Work out the finished part from the listing and answer in its coordinate system (mm). A direction names the side the tool comes from. Give positions to 0.01 mm unless a question says otherwise; leave off trailing zeros. Loops run counter-clockwise (first coordinate to the right, second up) from the corner with the lowest first, then second, coordinate; pieces in that order, holes last.
from build123d import *

# Parameters (mm, degrees)
IZIM2_R               = 8.5
KES_EKSTR_ZYON1_DEPTH = 89


with BuildPart() as part:
    # Çizim1 → Döndür1 (revolve)
    with BuildSketch(Plane.XY):
        Polygon((-44, 0), (-44, 12), (-41, 12), (-41, 11), (-40, 11), (-40, 12), (40, 12), (40, 11), (41, 11), (41, 12), (44, 12), (44, 0), align=None)
    revolve(axis=Axis((-44, 0, 0), (1, 0, 0)))

    # Çizim2 → Kes-Ekstrüzyon1 (cut, through all)
    with BuildSketch(Plane(origin=(44, 0, 0), x_dir=(0, 0, -1), z_dir=(1, 0, 0))):
        Circle(IZIM2_R)
    extrude(amount=-KES_EKSTR_ZYON1_DEPTH, mode=Mode.SUBTRACT)


solid = part.part
Item 1: Find section C-C, the plane x = 7.5. Write down the section's boundary in (y, z).
Item 2: Find section D-D, the plane z = 9.75. Write down the section's boundary in (x, y).
Item 3: Flat-ended cylindrical pins translate along their axes: pin 1 Ø8 at (y, z) = (-3.5, 3) entering from -X; pin 2 Ø10 at (x, z) = (-6.5, -5.5) entering from -Y; pin 3 Ø10 at (x, z) = (32.5, -8.5) entering from -Y; pin 4 Ø3 at (x, z) = (0.5, -7.5) entering from -Y. Find the tip coordinate at first contact, or state that the pin passes through.
Item 4: Consider line 1 (X direction, y = -10.5, z = 4.5); line 2 (Z direction, x = -16, y = -0.5); line 3 (Z direction, x = -36, y = 1.25). Determine where each line is inside the solid, lowest interval first.
Item 5: For faces 1 (the face through (40.51, -2.38, -10.74)), 2 (the face through (0.56, -11.99, 0.53)), determine the directions among +Z, -Z, +X, -X, +Y, -Y from which every point of the face is accessible in a straight line to the end or side of a thin tool.
Item 6: Find section A-A, the plane y = 0. Write down the section's boundary in (x, z).
Item 7: Determine the mould class of faces 3 (the face through (42.52, -11.99, 0.53)), 4 (the face through (44, -2.8, 8.2)), 5 (the face through (41, -5, -10)) for opening direction X: released by +X, released by -X, zero draft, split by the parting line, or undercut.
Ans:
1. outline: circle Ø24 at (0, 0); hole circle Ø17 at (0, 0)
2. outline: (-44, -7) - (-41, -7) - (-41, -5.09) - (-40, -5.09) - (-40, -7) - (40, -7) - (40, -5.09) - (41, -5.09) - (41, -7) - (44, -7) - (44, 7) - (41, 7) - (41, 5.09) - (40, 5.09) - (40, 7) - (-40, 7) - (-40, 5.09) - (-41, 5.09) - (-41, 7) - (-44, 7) - close
3. pin 1: stops at x = -44
3. pin 2: stops at y = -11.99
3. pin 3: stops at y = -11.48
3. pin 4: stops at y = -10.39
4. line 1: x = -44 to -41, -40 to 40, 41 to 44
4. line 2: z = -11.99 to -8.49, 8.49 to 11.99
4. line 3: z = -11.93 to -8.41, 8.41 to 11.93
5. face 1: none
5. face 2: +X, -X
6. outline: (-44, -12) - (-41, -12) - (-41, -11) - (-40, -11) - (-40, -12) - (40, -12) - (40, -11) - (41, -11) - (41, -12) - (44, -12) - (44, -8.5) - (-44, -8.5) - close; (-44, 8.5) - (44, 8.5) - (44, 12) - (41, 12) - (41, 11) - (40, 11) - (40, 12) - (-40, 12) - (-40, 11) - (-41, 11) - (-41, 12) - (-44, 12) - close
7. face 3: zero draft
7. face 4: released by +X
7. face 5: undercut
